```python
from build123d import *

# Parameters (mm, degrees)
F0_R     = 3
F0_R_2   = 1.4
F0_R_3   = 17.5
F0_R_4   = 1.5
F1_DEPTH = 3
F0_W     = 65
F0_H     = 3
F2_DEPTH = 67
F4_DEPTH = 136.001
F5_W     = 39.7
F5_H     = 3
F6_W     = 39.7
F6_H     = 3
F7_DEPTH = 5
F8_R     = 1
F9_R     = 5
F10_R    = 2


# Not quite as in the source:
# - a feature names something its author has since deleted; it is built from what else it names


with BuildPart() as f1:
    # F0 (on Top) → F1 (new body)
    with BuildSketch(Plane.XY):
        Polygon((-60.3749420391, 27.6098903269), (-60.3749420391, 7), (-15.3749420391, 7), (-15.3749420391, 12), (24.6250579609, 12), (24.6250579609, 7), (69.6250579609, 7), (69.6250579609, 53.4099719524), (69.6250579609, 87.5), (4.6250579609, 87.5), (-60.3749420391, 87.5), (-60.3749420391, 71.25), align=None)
        with Locations((-30.3749420391, 23.25)):
            Circle(F0_R, mode=Mode.SUBTRACT)
        with Locations((-11.3749420391, 31.25)):
            Circle(F0_R_2, mode=Mode.SUBTRACT)
        with Locations((20.6250579609, 31.25)):
            Circle(F0_R_2, mode=Mode.SUBTRACT)
        with Locations((52.6250579609, 23.25)):
            Circle(F0_R, mode=Mode.SUBTRACT)
        with Locations((-11.3749420391, 63.25)):
            Circle(F0_R_2, mode=Mode.SUBTRACT)
        with BuildLine():
            ThreePointArc((-27.3749420391, 71.25), (-30.3749420391, 68.25), (-33.3749420391, 71.25))
            ThreePointArc((-33.3749420391, 71.25), (-30.3749420391, 74.25), (-27.3749420391, 71.25))
        make_face(mode=Mode.SUBTRACT)
        with Locations((4.6250579609, 47.25)):
            Circle(F0_R_3, mode=Mode.SUBTRACT)
        with Locations((20.6250579609, 63.25)):
            Circle(F0_R_2, mode=Mode.SUBTRACT)
        with Locations((52.6250579609, 71.25)):
            Circle(F0_R, mode=Mode.SUBTRACT)
        Polygon((-15.3749420391, 12), (-15.3749420391, 7), (14.8769766092, 7), (24.6250579609, 7), (24.6250579609, 12), align=None)
        with BuildLine():
            ThreePointArc((-27.3749420391, 71.25), (-30.3749420391, 74.25), (-33.3749420391, 71.25))
            ThreePointArc((-33.3749420391, 71.25), (-30.3749420391, 68.25), (-27.3749420391, 71.25))
        make_face()
        with BuildLine():
            ThreePointArc((-28.8749420391, 71.25), (-30.3749420391, 69.75), (-31.8749420391, 71.25))
            ThreePointArc((-31.8749420391, 71.25), (-30.3749420391, 72.75), (-28.8749420391, 71.25))
        make_face(mode=Mode.SUBTRACT)
        with BuildLine():
            ThreePointArc((-28.8749420391, 71.25), (-30.3749420391, 72.75), (-31.8749420391, 71.25))
            ThreePointArc((-31.8749420391, 71.25), (-30.3749420391, 69.75), (-28.8749420391, 71.25))
        make_face()
        with Locations((52.6250579609, 71.25)):
            Circle(F0_R)
        with Locations((52.6250579609, 71.25)):
            Circle(F0_R_4, mode=Mode.SUBTRACT)
        with Locations((52.6250579609, 71.25)):
            Circle(F0_R_4)
        with Locations((52.6250579609, 23.25)):
            Circle(F0_R)
        with Locations((52.6250579609, 23.25)):
            Circle(F0_R_4, mode=Mode.SUBTRACT)
        with Locations((52.6250579609, 23.25)):
            Circle(F0_R_4)
        with Locations((-30.3749420391, 23.25)):
            Circle(F0_R)
        with Locations((-30.3749420391, 23.25)):
            Circle(F0_R_4, mode=Mode.SUBTRACT)
        with Locations((-30.3749420391, 23.25)):
            Circle(F0_R_4)
    extrude(amount=F1_DEPTH)

    # F0 (on Top) → F2 (join)
    with BuildSketch(Plane.XY):
        Polygon((-63.3749420391, 27.6098903269), (-60.3749420391, 27.6098903269), (-60.3749420391, 71.25), (-60.3749420391, 87.5), (-60.3749420391, 90.5), (-63.3749420391, 90.5), align=None)
        with Locations((-27.8749420391, 89)):
            Rectangle(F0_W, F0_H)
        with Locations((37.1250579609, 89)):
            Rectangle(F0_W, F0_H)
        Polygon((69.6250579609, 87.5), (69.6250579609, 53.4099719524), (72.6250579609, 53.4099719524), (72.6250579609, 90.5), (69.6250579609, 90.5), align=None)
        Polygon((69.6250579609, 7), (69.6250579609, 4), (72.6250579609, 4), (72.6250579609, 53.4099719524), (69.6250579609, 53.4099719524), align=None)
        Polygon((14.8769766092, 4), (69.6250579609, 4), (69.6250579609, 7), (24.6250579609, 7), (14.8769766092, 7), align=None)
        Polygon((-60.3749420391, 7), (-60.3749420391, 4), (14.8769766092, 4), (14.8769766092, 7), (-15.3749420391, 7), align=None)
        Polygon((-63.3749420391, 4), (-60.3749420391, 4), (-60.3749420391, 7), (-60.3749420391, 27.6098903269), (-63.3749420391, 27.6098903269), align=None)
    extrude(amount=F2_DEPTH)

    # F3 (on face) → F4 (cut, through all)
    with BuildSketch(Plane(origin=(-63.3749420391, 0, 0), x_dir=(0, -1, 0), z_dir=(-1, 0, 0))):
        with BuildLine():
            ThreePointArc((-20, 21.9706685841), (-12.9289321881, 24.8996007722), (-10, 31.9706685841))
            ThreePointArc((-10, 31.9706685841), (-20, 41.9706685841), (-30, 31.9706685841))
            ThreePointArc((-30, 31.9706685841), (-27.0710678119, 24.8996007722), (-20, 21.9706685841))
        make_face()
        with BuildLine():
            ThreePointArc((-30, 31.9706685841), (-20, 41.9706685841), (-10, 31.9706685841))
            Line((-10, 31.9706685841), (-10, 67))
            Line((-10, 67), (-30, 67))
            Line((-30, 67), (-30, 31.9706685841))
        make_face()
        with BuildLine():
            ThreePointArc((-74.5, 21.9706685841), (-67.4289321881, 24.8996007722), (-64.5, 31.9706685841))
            ThreePointArc((-64.5, 31.9706685841), (-74.5, 41.9706685841), (-84.5, 31.9706685841))
            ThreePointArc((-84.5, 31.9706685841), (-81.5710678119, 24.8996007722), (-74.5, 21.9706685841))
        make_face()
        with BuildLine():
            Line((-64.5, 31.9706685841), (-30, 31.9706685841))
            Line((-30, 31.9706685841), (-30, 67))
            Line((-30, 67), (-84.5, 67))
            Line((-84.5, 67), (-84.5, 31.9706685841))
            ThreePointArc((-84.5, 31.9706685841), (-74.5, 41.9706685841), (-64.5, 31.9706685841))
        make_face()
        with BuildLine():
            ThreePointArc((-20, 21.9706685841), (-27.0710678119, 24.8996007722), (-30, 31.9706685841))
            Line((-30, 31.9706685841), (-64.5, 31.9706685841))
            ThreePointArc((-64.5, 31.9706685841), (-67.4289321881, 24.8996007722), (-74.5, 21.9706685841))
            Line((-74.5, 21.9706685841), (-20, 21.9706685841))
        make_face()
    extrude(amount=-F4_DEPTH, mode=Mode.SUBTRACT)

    # F5 (on face) + F6 (on face) → F7 (join)
    with BuildSketch(Plane.XY.offset(67)):
        with Locations((4.6250579609, 5.5)):
            Rectangle(F5_W, F5_H)
    with BuildSketch(Plane.XY.offset(67)):
        with Locations((4.6250579609, 89)):
            Rectangle(F6_W, F6_H)
    extrude(amount=F7_DEPTH)

    # F8
    f8_edges = [f1.edges().sort_by_distance(p)[0] for p in [
        (-15.224942, 5.5, 67),
        (-15.224942, 5.5, 72),
        (24.475058, 5.5, 72),
        (24.475058, 5.5, 67),
        (-15.224942, 89, 67),
        (-15.224942, 89, 72),
        (24.475058, 89, 72),
        (24.475058, 89, 67),
    ]]
    fillet(f8_edges, radius=F8_R)

    # F9
    f9_edges = [f1.edges().sort_by_distance(p)[0] for p in [
        (72.625058, 4, 33.5),
        (72.625058, 90.5, 33.5),
        (-63.374942, 90.5, 33.5),
        (-63.374942, 4, 33.5),
        (-60.374942, 7, 35),
        (-60.374942, 87.5, 35),
        (69.625058, 87.5, 35),
        (69.625058, 7, 35),
    ]]
    fillet(f9_edges, radius=F9_R)

    # F10
    f10_edges = [f1.edges().sort_by_distance(p)[0] for p in [
        (4.625058, 87.5, 3),
        (4.625058, 4, 0),
    ]]
    fillet(f10_edges, radius=F10_R)


solid = f1.part
```
Check sheet for the modelled part. Datum: model origin and axes. Units: mm. A direction names the side the tool comes from. Round coordinates to 2 decimals unless told otherwise and drop trailing zeros. Loops run counter-clockwise (first coordinate to the right, second up) from the corner with the lowest first, then second, coordinate; pieces in that order, holes last. Notation, with made-up numbers: (88.25, 46) -> (105.25, 46) arc R28 ccw to (105.25, 84) -> close; hole circle Ø3 at (86, 46). An arc over 180 degrees is marked (long way). Answer in a Markdown table with one row per item.
Q1. Sectioned sample at D-D on x = 32. Enter the section's corners in (y, z).
Data:
| item | result |
|---|---|
| outline | (4, 2) arc R2 ccw to (6, 0) -> (88.5, 0) arc R2 ccw to (90.5, 2) -> (90.5, 67) -> (87.5, 67) -> (87.5, 5) arc R2 cw to (85.5, 3) -> (9, 3) arc R2 cw to (7, 5) -> (7, 67) -> (4, 67) -> close |
Q2. Thickness scan on L1, parallel to Y at x = 60, z = 39; L2, parallel to Z at x = 59, y = 10; L3, parallel to Y at x = -4.5, z = 4. Record the ranges inside material, lowest first.
Data:
| item | result |
|---|---|
| L1 | y = 4 to 7, 87.5 to 90.5 |
| L2 | z = 0 to 3 |
| L3 | y = 4 to 7.27, 87.23 to 90.5 |
Q3. Release check for a two-part mould opening along X. For faces 5 (the face through (2.35, 64.6, 1.48)), 6 (the face through (71, 84.5, 50)), 7 (the face through (-15.225, 89, 69)) record: released by +X, released by -X, zero draft, split by the parting line, or undercut.
Data:
| item | result |
|---|---|
| face 5 | undercut |
| face 6 | zero draft |
| face 7 | released by -X |
Q4. Set-up check for faces 1 (the face through (4, 65, 3)), 2 (the face through (71, 48, 21.971)), 3 (the face through (24.475, 5, 69)), 4 (the face through (-40, 6, 67)): record each of +Z, -Z, +X, -X, +Y, -Y from which the full face is reachable in a straight line by a thin tool's end or side.
Data:
| item | result |
|---|---|
| face 1 | +Z |
| face 2 | +Z, +X, -X |
| face 3 | +Z, +X, +Y, -Y |
| face 4 | +Z, -X, +Y, -Y |
Q5. Sectioned sample at B-B on z = 50. Enter the section's corners in (x, y).
Data:
| item | result |
|---|---|
| outline | (-63.37, 9) arc R5 ccw to (-58.37, 4) -> (67.63, 4) arc R5 ccw to (72.63, 9) -> (72.63, 10) -> (69.21, 10) arc R5 cw to (64.63, 7) -> (-55.37, 7) arc R5 cw to (-59.96, 10) -> (-63.37, 10) -> close; (-63.37, 84.5) -> (-59.96, 84.5) arc R5 cw to (-55.37, 87.5) -> (64.63, 87.5) arc R5 cw to (69.21, 84.5) -> (72.63, 84.5) -> (72.63, 85.5) arc R5 ccw to (67.63, 90.5) -> (-58.37, 90.5) arc R5 ccw to (-63.37, 85.5) -> close |
Q6. Sectioned sample at A-A on y = 47.25. Enter the section's corners in (x, z).
Data:
| item | result |
|---|---|
| outline | (-63.37, 2) arc R2 ccw to (-61.37, 0) -> (-12.87, 0) -> (-12.87, 3) -> (-58.37, 3) arc R2 cw to (-60.37, 5) -> (-60.37, 21.97) -> (-63.37, 21.97) -> close; (22.13, 0) -> (70.63, 0) arc R2 ccw to (72.63, 2) -> (72.63, 21.97) -> (69.63, 21.97) -> (69.63, 5) arc R2 cw to (67.63, 3) -> (22.13, 3) -> close |
Q7. Sectioned sample at C-C on x = 8.5. Enter the section's corners in (y, z), then the cut area to 3 significant figures.
Data:
| item | result |
|---|---|
| outline | (4, 2) arc R2 ccw to (6, 0) -> (30.18, 0) -> (30.18, 3) -> (9, 3) arc R2 cw to (7, 5) -> (7, 72) -> (4, 72) -> close; (64.32, 0) -> (88.5, 0) arc R2 ccw to (90.5, 2) -> (90.5, 72) -> (87.5, 72) -> (87.5, 5) arc R2 cw to (85.5, 3) -> (64.32, 3) -> close |
| area | 571 mm^2 |
Q8. Go/stop test with flat-tipped pins: P1, Ø3.5, axis at x = 71.5, y = 41, coming from the +Z side; P2, Ø2.5, axis at x = 70.5, z = 43.5, coming from the -Y side; P3, Ø3.5, axis at y = 89, z = 69.5, coming from the -X side; P4, Ø1, axis at x = 38.5, y = 75.5, coming from the -Z side. Record where each tip stops, or that it passes through.
Data:
| item | result |
|---|---|
| P1 | stops at z = 21.97 |
| P2 | stops at y = 4.27 |
| P3 | stops at x = -15.26 |
| P4 | stops at z = 0 |
